Work out the finished part from the listing and answer in its coordinate system (mm). A direction names the side the tool comes from. Give positions to 0.01 mm unless a question says otherwise; leave off trailing zeros. Order: outer loops, then holes, each group sorted by start corner. A loop starts at its lowest first (then second) coordinate and runs counter-clockwise, first axis right, second up. Notation, with made-up numbers: (57.5, 22.25) -> (87.5, 22.25) arc R18 cw to (87.5, 41.25) -> close; hole circle Ø7 at (70, 48.25). An arc over 180 degrees is marked (long way). Answer as CSV lines item,"result". Start each with the question number.
1. A cutting plane is placed at C-C (y = 57.5). Give the vertices of the cut face in (x, z), then the cut area to 3 significant figures.
2. Flat-ended cylindrical pins translate along their axes: pin 1 (2 mm diameter, centred on y = 34.5, z = 3, fed in from +X); pin 2 (3 mm diameter, centred on x = -6, z = 4.5, fed in from -Y); pin 3 (1 mm diameter, centred on y = 7.5, z = 2.5, fed in from +X). Find the tip coordinate at first contact, or state that the pin passes through.
3. A cutting plane is placed at B-B (x = 1.5). Give the vertices of the cut face in (y, z), then the cut area to 3 significant figures.
4. For a pull along Y with two mould halves and no side action, classify faces 1 (the cylindrical face through (31.293, 59.344, 2.958)), 2 (the flat face through (0, 66, 0)), 3 (the cylindrical face through (0.09, -6.05, 2.96)), 4 (the flat face through (-19.665, 20.867, 2.958)) as released by +Y, released by -Y, zero draft, split by the parting line, or undercut.
5. Find the intervals of material crossed by L1, parallel to Y at x = 0, z = 0.7; L2, parallel to Y at x = -6, z = 2.9; L3, parallel to X at y = 46, z = 3, in increasing order.
6. A cutting plane is placed at A-A (z = 1.6). Give the vertices of the cut face in (x, y).
7. For faces 5 (the flat face through (0, 66.85, 3)), 6 (the cylindrical face through (-31.5, 59, 3)), determine the directions among +Z, -Z, +X, -X, +Y, -Y from which every point of the face is accessible in a straight line to the end or side of a thin tool.
Autodesk Inventor part; units mm, degrees
ref_plane "YZ Plane" through (0, 0, 0) normal (1, 0, 0) x (0, 1, 0)
ref_plane "XZ Plane" through (0, 0, 0) normal (0, 1, 0) x (-1, 0, 0)
ref_plane "XY Plane" through (0, 0, 0) normal (0, 0, 1) x (1, 0, 0)
sketch "Sketch1" plane through (0, 0, 0) normal (0, 0, 1) x (1, 0, 0)
  arc A0 (-5.3402, -2.8434) -> (5.3402, -2.8434) centre (0, 0) ccw
  arc A1 (-6.6642, -3.5484) -> (6.6642, -3.5484) centre (0, 0) ccw
  circle A2 centre (-20.5, 52.65) radius 1.25
  circle A3 centre (20.5, 52.65) radius 1.25
  arc A4 (-20.5, 65.35) -> (-31.71, 46.6812) centre (-20.5, 52.65) ccw
  arc A5 (31.71, 46.6812) -> (20.5, 65.35) centre (20.5, 52.65) ccw
  arc A6 (-20.5, 66.85) -> (-33.034, 45.9762) centre (-20.5, 52.65) ccw
  arc A7 (33.034, 45.9762) -> (20.5, 66.85) centre (20.5, 52.65) ccw
  line L0 (-6.6642, -3.5484) -> (-33.034, 45.9762)
  line L1 (-31.71, 46.6812) -> (-5.3402, -2.8434)
  line L2 (6.6642, -3.5484) -> (33.034, 45.9762)
  line L3 (5.3402, -2.8434) -> (31.71, 46.6812)
  line L4 (-20.5, 66.85) -> (20.5, 66.85)
  line L5 (20.5, 65.35) -> (-20.5, 65.35)
  dimension "d0" = 12.1
  dimension "d4" = 25.4
  dimension "d5" = 25.4
  dimension "d6" = 1.5
  dimension "d7" = 1.5
extrude "Extrusion1" add sketch "Sketch1" along normal blind 6 contours L0 A6 L4 A7 L2 A1
equation "\"d4\" = d5"
properties part number "Belt_A" material "Rubber"
Answer sheet:
1,outline,"(-33.85, 0) -> (-32.24, 0) -> (-32.24, 6) -> (-33.85, 6) -> close; (32.24, 0) -> (33.85, 0) -> (33.85, 6) -> (32.24, 6) -> close"
1,area,"19.3 mm^2"
2,pin 1,"stops at x = 27.46"
2,pin 2,"stops at y = -6.06"
2,pin 3,"stops at x = 12.81"
3,outline,"(-7.4, 0) -> (-5.86, 0) -> (-5.86, 6) -> (-7.4, 6) -> close; (65.35, 0) -> (66.85, 0) -> (66.85, 6) -> (65.35, 6) -> close"
3,area,"18.2 mm^2"
4,face 1,"undercut"
4,face 2,"zero draft"
4,face 3,"undercut"
4,face 4,"released by -Y"
5,L1,"y = -7.55 to -6.05, 65.35 to 66.85"
5,L2,"y = -4.58 to -1.6, 65.35 to 66.85"
5,L3,"x = -33.05 to -31.35, 31.35 to 33.05"
6,outline,"(-33.03, 45.98) -> (-6.66, -3.55) arc R7.55 ccw to (6.66, -3.55) -> (33.03, 45.98) arc R14.2 ccw to (20.5, 66.85) -> (-20.5, 66.85) arc R14.2 ccw to start; hole (-31.71, 46.68) -> (-5.34, -2.84) arc R6.05 ccw to (5.34, -2.84) -> (31.71, 46.68) arc R12.7 ccw to (20.5, 65.35) -> (-20.5, 65.35) arc R12.7 ccw to start"
7,face 5,"+Z, -Z, +X, -X, +Y"
7,face 6,"+Z, -Z"
